from build123d import *
from build123d.topology import SkipClean

# Parameters (mm, degrees)
SKETCH1_W           = 38.452994616
SKETCH1_H           = 5
BOSS_EXTRUDE1_DEPTH = 75
BOSS_EXTRUDE2_START = -10
BOSS_EXTRUDE2_DEPTH = 55
SKETCH5_R           = 3.175
CUT_EXTRUDE8_DEPTH  = 55
CUT_EXTRUDE9_DEPTH  = 75
CUT_EXTRUDE10_DEPTH = 10
CUT_EXTRUDE11_START = -65
CUT_EXTRUDE11_DEPTH = 10


with BuildPart() as part:
    # Sketch1 → Boss-Extrude1 (new body)
    with BuildSketch(Plane.XY):
        with Locations((25, -2.5)):
            Rectangle(SKETCH1_W, SKETCH1_H)
    extrude(amount=-BOSS_EXTRUDE1_DEPTH)

    # Sketch1_4 → Boss-Extrude2 (add)
    with BuildSketch(Plane.XY.offset(BOSS_EXTRUDE2_START)):
        with BuildLine():
            ThreePointArc((10.773502692, -5), (9.309036598, -1.464466094), (5.773502692, 0))
            Line((5.773502692, 0), (5.773502692, -2.5))
            ThreePointArc((5.773502692, -2.5), (7.541269645, -3.232233047), (8.273502692, -5))
            Line((8.273502692, -5), (10.773502692, -5))
        make_face()
        with BuildLine():
            Line((5.773502692, -2.5), (5.773502692, 0))
            ThreePointArc((5.773502692, 0), (3.273502704, -0.669872974), (1.443375686, -2.499999977))
            ThreePointArc((1.443375686, -2.499999977), (4.479407453, -9.829629128), (10.773502692, -5))
            Line((10.773502692, -5), (8.273502692, -5))
            ThreePointArc((8.273502692, -5), (4.005735739, -6.767766953), (5.773502692, -2.5))
        make_face()
    extrude(amount=-BOSS_EXTRUDE2_DEPTH)

    # Sketch5 → Cut-Extrude8 (cut)
    with BuildSketch(Plane.XZ.offset(5)):
        with Locations((25, -25)):
            Circle(SKETCH5_R)
        with Locations((25, -50)):
            Circle(SKETCH5_R)
    extrude(amount=-CUT_EXTRUDE8_DEPTH, mode=Mode.SUBTRACT)

    # Sketch1_14 → Cut-Extrude9 (cut)
    with SkipClean():  # the faces are left unmerged after this step: merging them gives an invalid solid
        with BuildSketch(Plane.XY):
            with BuildLine():
                ThreePointArc((8.273502692, -5), (7.541269645, -3.232233047), (5.773502692, -2.5))
                Line((5.773502692, -2.5), (5.773502692, -5))
                Line((5.773502692, -5), (8.273502692, -5))
            make_face()
            with BuildLine():
                Line((5.773502692, -5), (5.773502692, -2.5))
                ThreePointArc((5.773502692, -2.5), (4.005735739, -6.767766953), (8.273502692, -5))
                Line((8.273502692, -5), (5.773502692, -5))
            make_face()
        extrude(amount=-CUT_EXTRUDE9_DEPTH, mode=Mode.SUBTRACT)

    # Sketch1_15 → Cut-Extrude10 (cut)
    with BuildSketch(Plane.XY):
        with BuildLine():
            ThreePointArc((10.773502692, -5), (9.309036598, -1.464466094), (5.773502692, 0))
            Line((5.773502692, 0), (5.773502692, -2.5))
            ThreePointArc((5.773502692, -2.5), (7.541269645, -3.232233047), (8.273502692, -5))
            Line((8.273502692, -5), (10.773502692, -5))
        make_face()
        with BuildLine():
            Line((5.773502692, -2.5), (5.773502692, 0))
            ThreePointArc((5.773502692, 0), (3.273502704, -0.669872974), (1.443375686, -2.499999977))
            ThreePointArc((1.443375686, -2.499999977), (4.479407453, -9.829629128), (10.773502692, -5))
            Line((10.773502692, -5), (8.273502692, -5))
            ThreePointArc((8.273502692, -5), (4.005735739, -6.767766953), (5.773502692, -2.5))
        make_face()
    extrude(amount=-CUT_EXTRUDE10_DEPTH, mode=Mode.SUBTRACT)

    # Sketch1_16 → Cut-Extrude11 (cut)
    with BuildSketch(Plane.XY.offset(CUT_EXTRUDE11_START)):
        with BuildLine():
            ThreePointArc((10.773502692, -5), (9.309036598, -1.464466094), (5.773502692, 0))
            Line((5.773502692, 0), (5.773502692, -2.5))
            ThreePointArc((5.773502692, -2.5), (7.541269645, -3.232233047), (8.273502692, -5))
            Line((8.273502692, -5), (10.773502692, -5))
        make_face()
        with BuildLine():
            Line((5.773502692, -2.5), (5.773502692, 0))
            ThreePointArc((5.773502692, 0), (3.273502704, -0.669872974), (1.443375686, -2.499999977))
            ThreePointArc((1.443375686, -2.499999977), (4.479407453, -9.829629128), (10.773502692, -5))
            Line((10.773502692, -5), (8.273502692, -5))
            ThreePointArc((8.273502692, -5), (4.005735739, -6.767766953), (5.773502692, -2.5))
        make_face()
    extrude(amount=-CUT_EXTRUDE11_DEPTH, mode=Mode.SUBTRACT)


solid = part.part
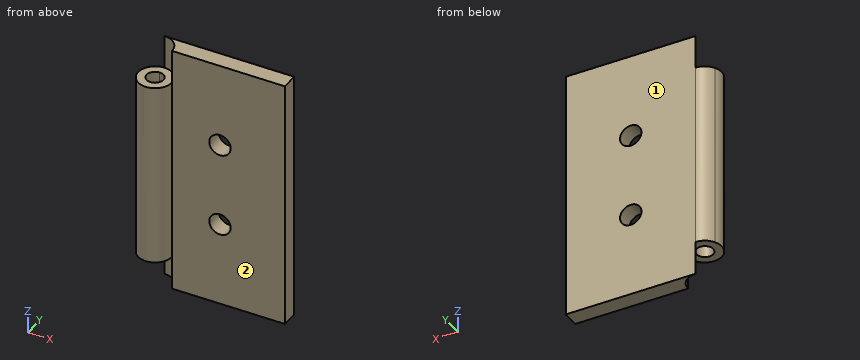
Design review of the part built by this model. Coordinates are the model's own, in mm. Face numbers are marked on the shaded views. A direction names the side the tool comes from. Round coordinates to 2 decimals unless told otherwise and drop trailing zeros. Write each loop counter-clockwise with the first axis right and the second up, starting at its lowest first coordinate (ties: lowest second). Pieces come first, ordered by that corner, then holes. Notation, with made-up numbers: (-4, -21.5) -> (3, -21.5) arc R20 ccw to (3, 14.5) -> close; hole circle Ø3 at (43.5, -39). An arc over 180 degrees is marked (long way). One line per item, written item: value. Start each with the question number.
Q1. Add section A-A (z = -25). Give the boundary of the cut face in (x, y) (1 decimal).
Q2. Add section C-C (x = 25). Give the boundary of the cut face in (y, z) (3 decimals), then the cut area to 4 significant figures.
Q3. To check wall thickness, follow probe 1 along Z at (x, y) = (25, -2) (3 decimals); probe 2 along Y at (x, z) = (5.5, -47) (3 decimals); probe 3 along Y at (x, z) = (35, -12). State the ranges of each line that lie inside material, in increasing order.
Q4. Tool access review of the marked faces 1 and 2: name each direction out of +Z, -Z, +X, -X, +Y, -Y from which nothing blocks a thin tool from reaching the whole face with its end or side.
Q5. Add section B-B (z = -56). Give the boundary of the cut face in (x, y), then the cut area to 3 significant figures.
Q6. Add section D-D (y = -0.75). State how many separate pieces and enclosed holes the cut face has, then the cut area to 3 significant figures.
Q7. Insertion check: P1, Ø1, axis at y = -7.5, z = -22, coming from the +X side; P2, Ø8.5, axis at x = 25, z = -25, coming from the -Y side; P3, Ø12, axis at x = 33, z = -12, coming from the +Y side; P4, Ø3, axis at x = 5, y = -4, coming from the +Z side. Each pin has a flat end and moves straight along its axis. Give the tip position at first contact, or say it passes through.
Response:
1. outline: (5.8, 0) arc R5 ccw (long way) to (10.8, -5) -> (21.8, -5) -> (21.8, 0) -> close; (28.2, -5) -> (44.2, -5) -> (44.2, 0) -> (28.2, 0) -> close; hole circle Ø5 at (5.8, -5)
2. outline: (-5, -75) -> (0, -75) -> (0, -53.175) -> (-5, -53.175) -> close; (-5, -46.825) -> (0, -46.825) -> (0, -28.175) -> (-5, -28.175) -> close; (-5, -21.825) -> (0, -21.825) -> (0, 0) -> (-5, 0) -> close
2. area: 311.5 mm^2
3. probe 1: z = -75 to -53.175, -46.825 to -28.175, -21.825 to 0
3. probe 2: y = -9.993 to -7.485, -2.515 to -0.007
3. probe 3: y = -5 to 0
4. face 1: +Z, -Z, +X, -X, +Y
4. face 2: +Z, -Z, +X, -Y
5. outline: (5.77, 0) arc R5 ccw (long way) to (10.77, -5) -> (44.23, -5) -> (44.23, 0) -> close; hole circle Ø5 at (5.77, -5)
5. area: 232 mm^2
6. separate pieces: 1
6. enclosed holes: 2
6. area: 2,910 mm^2
7. P1: stops at x = 10.36
7. P2: stops at y = -5
7. P3: stops at y = 0
7. P4: stops at z = -10
